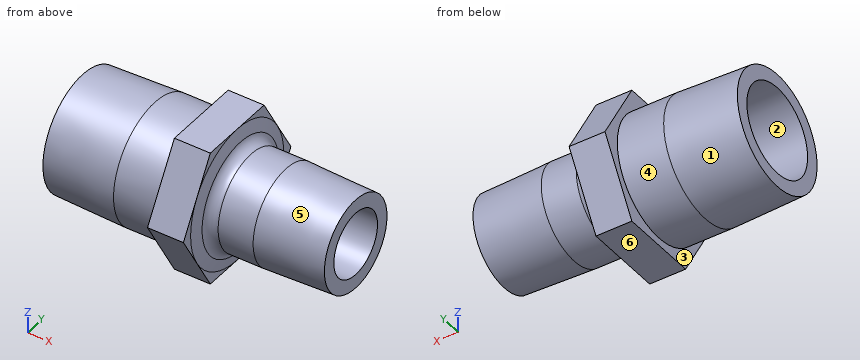
Autodesk Inventor part; units mm, degrees
ref_plane "Work Plane1" through (19, 0, 0) normal (1, 0, 0) x (0, 1, 0)
ref_plane "YZ Plane" through (0, 0, 0) normal (1, 0, 0) x (0, 1, 0)
ref_plane "XZ Plane" through (0, 0, 0) normal (0, 1, 0) x (-1, 0, 0)
sketch "Sketch1" plane through (0, 0, 0) normal (0, 0, 1) x (1, 0, 0)
  line L0 (0, 0) -> (38, 0)
  line L1 (0, 0) -> (0, 6.2) construction
  line L2 (19, 4.45) -> (19, 6.2)
  line L3 (38, 4.45) -> (38, 0) construction
  line L4 (0, 6.2) -> (0, 8.1326)
  line L5 (38, 4.45) -> (38, 6.3907)
  line L6 (28.29, 6.6941) -> (28.29, 0) construction
  line L7 (16.5, 9.5) -> (21.5, 9.5)
  line L8 (19, 6.2) -> (19, 9.5) construction
  line L9 (19, 6.2) -> (0, 6.2)
  line L10 (19, 4.45) -> (38, 4.45)
  line L11 (0, 8.1326) -> (10.05, 8.4466)
  line L12 (10.05, 8.4466) -> (10.05, 0) construction
  line L13 (10.05, 8.4466) -> (16.5, 8.4466)
  line L14 (16.5, 8.4466) -> (16.5, 9.5)
  line L15 (38, 6.3907) -> (28.29, 6.6941)
  line L16 (21.5, 6.6941) -> (21.5, 9.5) construction
  line L17 (19, 4.45) -> (19, 0) construction
  line L18 (21.5, 9.5) -> (21.9504, 7.8192)
  line L19 (28.29, 6.6941) -> (23.4166, 6.6941)
  line L20 (21.5, 6.6941) -> (23.4166, 6.6941) construction
  arc A0 (21.9504, 7.8192) -> (23.4166, 6.6941) centre (23.4166, 8.2121) ccw
  line L21 (6.35, 8.331) -> (6.35, 0) construction
  line L22 (31.99, 6.5785) -> (31.99, 0) construction
  dimension "d0" = 38
  dimension "d3" = 19
  dimension "d4" = 19
  dimension "d5" = 8.9
  dimension "d7" = 1.79
  dimension "d8" = 12.4
  dimension "d10" = 1.79
  dimension "d11" = 10.05
  dimension "d12" = 5
  dimension "d13" = 9.71
  dimension "d18" = 15
  dimension "d23" = 1.518
  dimension "d27" = 6.35
  dimension "d28" = 6.01
  dimension "d29" = 16.662
  dimension "d30" = 13.157
revolve "Revolve1" add sketch "Sketch1" angle 360 about axis through (0, 0, 0) along (1, 0, 0)
ref_plane "Work Plane1" through (19, 0, 0) normal (1, 0, 0) x (0, 1, 0)
sketch "Sketch2" plane through (19, 0, 0) normal (1, 0, 0) x (0, 1, 0)
  circle A0 centre (0, 0) radius 9.5
  line L0 (-5.4848, -9.5) -> (-10.9697, 0)
  line L1 (-10.9697, 0) -> (-5.4848, 9.5)
  line L2 (-5.4848, 9.5) -> (5.4848, 9.5)
  line L3 (5.4848, 9.5) -> (10.9697, 0)
  line L4 (10.9697, 0) -> (5.4848, -9.5)
  line L5 (5.4848, -9.5) -> (-5.4848, -9.5)
  point P0 (0, 0)
  point P1 (0, 0)
  point P2 (0, -9.5)
extrude "Extrude1" add sketch "Sketch2" along normal mid plane 5 contours A0 L3 L4 | A0 L2 L3 | L4 L5 A0 | A0 L1 L2 | L5 L0 A0 | A0 L0 L1
thread "Gwint1"
thread "Gwint2"
equation "\"d0\" = a"
equation "\"d3\" = 0.5 * a"
equation "\"d4\" = S"
equation "\"d5\" = d2"
equation "\"d8\" = d1"
equation "\"d11\" = L1"
equation "\"d12\" = M"
equation "\"d13\" = L2"
equation "\"d23\" = 0.11 * OD2"
equation "\"d27\" = a1"
equation "\"d28\" = a2"
equation "\"d29\" = DD1"
equation "\"d30\" = DD2"
equation "\"d16\" = M"
equation "\"OD1\" = 17.3"
equation "\"OD2\" = 13.8"
equation "\"a\" = 38"
equation "\"d1\" = 12.4"
equation "\"d2\" = 8.9"
equation "\"M\" = 5"
equation "\"S\" = 19"
equation "\"L1\" = 10.05"
equation "\"L2\" = 9.71"
equation "\"d14\" = 0.5 * a"
equation "\"a1\" = 6.35"
equation "\"DD1\" = 16.662"
equation "\"a2\" = 6.01"
equation "\"DD2\" = 13.157"
equation "\"Size_Designation\" = 1.2345"
properties part number "ISO 49 Złączka wkrętna sześciokątna, redukcyjna N8 3/8 x 1/4" material "Żelazo, ciągliwe"
CAD build for the part. Positions are in the model's coordinates, mm. Face numbers are marked on the shaded views. A direction names the side the tool comes from. Round coordinates to 2 decimals unless told otherwise and drop trailing zeros. Write each loop counter-clockwise with the first axis right and the second up, starting at its lowest first coordinate (ties: lowest second). Pieces come first, ordered by that corner, then holes. Notation, with made-up numbers: (21.25, -20) - (34.25, -20) arc R25 ccw to (34.25, -6) - close; hole circle Ø10 at (69.5, 54). An arc over 180 degrees is marked (long way). Write item = value, one per line. Start each with the question number.
Q1. Drop flat-ended pins along their axis: pin 1 (2 mm diameter, centred on x = 17, z = -5.5, fed in from +Y); pin 2 (4 mm diameter, centred on y = -5.5, z = 8, fed in from +X); pin 3 (5 mm diameter, centred on x = 12.5, z = -1.5, fed in from -Y); pin 4 (7.5 mm diameter, centred on y = 0, z = 0, fed in from +X). Give the stop position or say it passes through.
Q2. Mould opens along Y. For the marked faces 1, 2 and 3 say: pulls with the +Y half, pulls with the -Y half, needs draft (parallel to the pull), parting line crosses it, or undercut.
Q3. Band-saw the part on B-B (x = 30). Give the cut face in (y, z), then the cut area to 3 significant figures.
Q4. Probe L1, parallel to Z at x = 28.25, y = 0; L2, parallel to X at y = 2.5, z = 5.5; L3, parallel to Y at x = 32, z = -1.75. List the from-to ranges inside material, lowest first. Write a range as from..to.
Q5. Which spindle directions (+Z, -Z, +X, -X, +Y, -Y) get a long thin tool onto all of the face, cutting with end or side? Do the marked faces 4, 5 and 6. Say none if no direction does.
Q6. Band-saw the part on A-A (x = 10.5). Give the cut face in (y, z).
Answers below:
q1.pin_1 = 8.37
q1.pin_2 = 21.98
q1.pin_3 = -8.45
q1.pin_4 = through
q2.face_1 = parting line crosses it
q2.face_2 = undercut
q2.face_3 = needs draft
q3.outline = circle Ø13.28 at (0, 0); hole circle Ø8.9 at (0, 0)
q3.area = 76.3 mm2
q4.L1 = -6.69..-4.45, 4.45..6.69
q4.L2 = 19..38
q4.L3 = -6.34..-4.09, 4.09..6.34
q5.face_4 = -X
q5.face_5 = +X
q5.face_6 = -Z, +X, -X, +Y, -Y
q6.outline = circle Ø16.89 at (0, 0); hole circle Ø12.4 at (0, 0)
